```python
from build123d import *

# Parameters (mm, degrees)
F1_DEPTH = 25


with BuildPart() as f1:
    # F0 (on Top) → F1 (new body)
    with BuildSketch(Plane.XY):
        Polygon((72.5, 70), (72.5, 75), (-72.5, 75), (-72.5, 70), (-69.5, 70), (-69.5, 65), (-72.5, 65), (-72.5, 60), (-69.5, 60), (-69.5, 55), (-72.5, 55), (-72.5, 50), (-69.5, 50), (-69.5, 45), (-72.5, 45), (-72.5, 40), (-69.5, 40), (-69.5, 35), (-72.5, 35), (-72.5, 30), (-69.5, 30), (-69.5, 25), (-72.5, 25), (-72.5, 20), (-69.5, 20), (-69.5, 15), (-72.5, 15), (-72.5, 10), (-69.5, 10), (-69.5, 5), (-72.5, 5), (-72.5, 0), (-72.5, -5), (-69.5, -5), (-69.5, -10), (-72.5, -10), (-72.5, -15), (-69.5, -15), (-69.5, -20), (-72.5, -20), (-72.5, -25), (-69.5, -25), (-69.5, -30), (-72.5, -30), (-72.5, -35), (-69.5, -35), (-69.5, -40), (-72.5, -40), (-72.5, -45), (-69.5, -45), (-69.5, -50), (-72.5, -50), (-72.5, -55), (-69.5, -55), (-69.5, -60), (-72.5, -60), (-72.5, -65), (-69.5, -65), (-69.5, -70), (-72.5, -70), (-72.5, -75), (72.5, -75), (72.5, -70), (69.5, -70), (69.5, -65), (72.5, -65), (72.5, -60), (69.5, -60), (69.5, -55), (72.5, -55), (72.5, -50), (69.5, -50), (69.5, -45), (72.5, -45), (72.5, -40), (69.5, -40), (69.5, -35), (72.5, -35), (72.5, -30), (69.5, -30), (69.5, -25), (72.5, -25), (72.5, -20), (69.5, -20), (69.5, -15), (72.5, -15), (72.5, -10), (69.5, -10), (69.5, -5), (72.5, -5), (72.5, 0), (72.5, 5), (69.5, 5), (69.5, 10), (72.5, 10), (72.5, 15), (69.5, 15), (69.5, 20), (72.5, 20), (72.5, 25), (69.5, 25), (69.5, 30), (72.5, 30), (72.5, 35), (69.5, 35), (69.5, 40), (72.5, 40), (72.5, 45), (69.5, 45), (69.5, 50), (72.5, 50), (72.5, 55), (69.5, 55), (69.5, 60), (72.5, 60), (72.5, 65), (69.5, 65), (69.5, 70), align=None)
    extrude(amount=F1_DEPTH)


solid = f1.part
```
Could you check a few things on this model? Use its own coordinates, in mm. A direction names the side the tool comes from. Round coordinates to 2 decimals unless told otherwise and drop trailing zeros. Loops run counter-clockwise (first coordinate to the right, second up) from the corner with the lowest first, then second, coordinate; pieces in that order, holes last. Notation, with made-up numbers: M 24,25.5 L 66,25.5 A19 ccw 66,53.5 Z; hole C 45,-11.75 d10. An arc over 180 degrees is marked long. Answer as CSV lines item,"result".
1) Which directions (+Z, -Z, +X, -X, +Y, -Y) give clear straight access to the entire face, cutting with the end or side of a thin tool? Please do faces 4 (the flat face through (69.5, -28, 12)), 5 (the flat face through (-72.5, -32, 12)), 6 (the flat face through (-69.5, -57, 12)).
From the geometry:
face 4,"+Z, -Z, +X"
face 5,"+Z, -Z, -X, +Y, -Y"
face 6,"+Z, -Z, -X"
2) For pin 1 Ø1.5 at (y, z) = (-58.5, 11) entering from +X; pin 2 Ø1.5 at (y, z) = (-68.5, 12) entering from -X, each with a flat end and sliding along its axis, tell me the tip position at first contact or that it passes through.
From the geometry:
pin 1,"x = 69.5"
pin 2,"x = -69.5"
3) If I drill on probe 1 along X at (y, z) = (-47.5, 14), over which ranges is the centre line in solid material (lowest first)?
From the geometry:
probe 1,"-69.5 to 69.5"
4) Imagine slicing it at A-A on y = -27.5. List the corners of the cut face in (x, z) for me.
From the geometry:
outline,"M -69.5,0 L 69.5,0 L 69.5,25 L -69.5,25 Z"
5) We'd pull the mould along Y, two halves only. Please class faces 1 (the flat face through (1, 75, 12)), 2 (the flat face through (-72.5, 73, 12)), 3 (the flat face through (69.5, 17, 12)): released by +Y, released by -Y, zero draft, split by the parting line, or undercut.
From the geometry:
face 1,"released by +Y"
face 2,"zero draft"
face 3,"undercut"
